Input: part model. Units: mm. Frame: model coordinates. Face numbers are marked on the shaded views. Give positions to 0.01 mm unless a question says otherwise; leave off trailing zeros. Loops run counter-clockwise (first coordinate to the right, second up) from the corner with the lowest first, then second, coordinate; pieces in that order, holes last. Notation, with made-up numbers: M -38,19.5 L -5,19.5 A33 ccw -5,49.5 Z; hole C 57.25,1.5 d1. An arc over 180 degrees is marked long. Answer as a JSON object with one key per item and string values. Group by question number.
1) Section query C-C on y = -0.85. Count the separate pieces of the cut face and the enclosed holes in it, plus the area to 3 significant figures.
2) Draft query along Z for the marked faces 1 and 2. Return one class per face: +Z half, -Z half, draft (parallel to the pull), parting line (faces both ways), or undercut.
3) Ray query, L1, parallel to Z at x = -40, y = 0; L2, parallel to X at y = -1.35, z = 15; L3, parallel to Z at x = 58, y = 0.2. Return the intervals inside material, ascending.
4) First-contact query: P1, Ø2.5, axis at y = 1, z = 22.5, coming from the -X side; P2, Ø1, axis at x = -36.5, y = -1, coming from the +Z side; P3, Ø2.5, axis at x = -57.5, y = 0.5, coming from the +Z side; P4, Ø1, axis at x = 47, z = -26, coming from the -Y side. Flat tips, straight axial feed; report the tip coordinate or a pass-through.
5) Section query B-B on x = -15. Return loops of the section in (y, z).
6) Section query A-A on z = 0. Return loops of the section in (x, y), plus the area to 3 significant figures.
from build123d import *

# Parameters (mm, degrees)
F1_DEPTH  = 2.5
F2_T      = -2
F5_SIZE   = 1
F6_W      = 75
F6_H      = 5
F7_DEPTH  = 37.501
F8_W      = 2
F8_H      = 7.2075595917
F9_DEPTH  = 6
F12_R     = 5
F13_DEPTH = 5
F15_D     = 6


with BuildPart() as f1:
    # F0 (on Front) → F1 (new body, symmetric)
    with BuildSketch(Plane.XZ):
        with BuildLine():
            Line((0, 10), (0, 0))
            Line((0, 0), (70, 0))
            Line((70, 0), (70, 10))
            Line((70, 10), (50, 10))
            ThreePointArc((50, 10), (46.4644660941, 11.4644660941), (45, 15))
            Line((45, 15), (45, 25))
            Line((45, 25), (35, 25))
            Line((35, 25), (35, 15))
            ThreePointArc((35, 15), (33.5355339059, 11.4644660941), (30, 10))
            Line((30, 10), (0, 10))
        make_face()
    extrude(amount=F1_DEPTH, both=True)

    # F2
    f2_openings = [f1.faces().sort_by_distance(p)[0] for p in [
        (35.933685, -2.5, 7.254637),
    ]]
    offset(amount=F2_T, openings=f2_openings)

    # F3 (on Front) → F4 (revolve)
    with BuildSketch(Plane.XZ):
        Polygon((37, 25), (40, 25), (40, 37.5), (37, 37.5), (37, 35.5), (37.5, 35.5), (37.5, 27), (37, 27), align=None)
    revolve(axis=Axis((40, 0, 31.25), (0, 0, 1)))

    # F5
    f5_edges = [f1.edges().sort_by_distance(p)[0] for p in [
        (43, 0, 37.5),
    ]]
    chamfer(f5_edges, length=F5_SIZE)

    # F6 (on face) → F7 (intersect, through all)
    with BuildSketch(Plane.XY.offset(37.5)):
        with Locations((35.0987253711, 0)):
            Rectangle(F6_W, F6_H)
    extrude(amount=-F7_DEPTH, mode=Mode.INTERSECT)

    # F8 (on face) → F9 (cut)
    with BuildSketch(Plane.XY.offset(37.5)):
        with Locations((40, -0.078830868)):
            Rectangle(F8_W, F8_H)
    extrude(amount=-F9_DEPTH, mode=Mode.SUBTRACT)

    # F10: F1 across face


with BuildPart() as f1_1:
    add(f1.part)
    add(f1.part.mirror(Plane(origin=(35, 0, 0), x_dir=(1, 0, 0), z_dir=(0, 0, -1))))

    # F11: F1 across face


with BuildPart() as f1_2:
    add(f1_1.part)
    add(f1_1.part.mirror(Plane(origin=(0, 0, 0), x_dir=(0, -1, 0), z_dir=(-1, 0, 0))))

    # F12 (on face) → F13 (join, through all)
    with BuildSketch(Plane.XZ.offset(2.5)):
        with Locations((-40, 0)):
            Circle(F12_R)
        with Locations((-15, 0)):
            Circle(F12_R)
    extrude(amount=-F13_DEPTH)

    # F15 (through all)
    with Locations(Plane.XZ.offset(2.5)):
        with Locations((-40, 0), (-15, 0)):
            Hole(F15_D / 2)


solid = f1_2.part
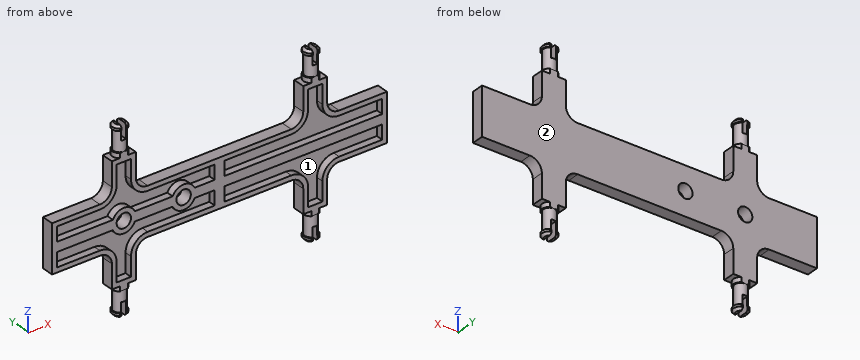
Output:
{
 "1": {"separate pieces": "1", "enclosed holes": "6", "area": "1,640 mm^2"},
 "2": {"face 1": "undercut", "face 2": "draft"},
 "3": {"L1": "z = -31.5 to -23, -5 to -3, 3 to 5, 23 to 31.5", "L2": "x = -45 to -43, -37 to -35, 35 to 37, 43 to 45", "L3": "z = -10 to -8, -2 to 2, 8 to 10"},
 "4": {"P1": "stops at x = -45", "P2": "stops at z = 25", "P3": "stops at z = 10", "P4": "passes through"},
 "5": {"outline": "M -2.5,-10 L 2.5,-10 L 2.5,-3 L -2.5,-3 L -2.5,-5 L 0.5,-5 L 0.5,-8 L -2.5,-8 Z; M -2.5,3 L 2.5,3 L 2.5,10 L -2.5,10 L -2.5,8 L 0.5,8 L 0.5,5 L -2.5,5 Z"},
 "6": {"outline": "M -70,-2.5 L -43,-2.5 L -43,2.5 L -70,2.5 Z; M -37,-2.5 L -18,-2.5 L -18,2.5 L -37,2.5 Z; M -12,-2.5 L 70,-2.5 L 70,2.5 L -12,2.5 Z", "area": "640 mm^2"}
}
